Input: dimensioned drawing with shaded views. Units: mm. Origin: part minimum x, y, z. Give positions to 0.01 mm unless a question says otherwise; leave off trailing zeros. Order: outer loops, then holes, each group sorted by start corner. A loop starts at its lowest first (then second) coordinate and runs counter-clockwise, first axis right, second up. Notation, with made-up numbers: M 55.5,2.5 L 60.5,2.5 A7 ccw 60.5,14.5 Z; hole C -22,-38.75 d5. An arc over 180 degrees is marked long. Answer in a Markdown table with one row per item. Add a question column.
(1) Section query B-B, the plane x = 4.85. Return loops of the section in (y, z).
(2) Material intervals for line 1 along Y through (x, z) = (5, 1.7); line 2 along Y through (x, z) = (8.25, 1.45); line 3 along X through (y, z) = (25.5, 2.3), sorted ascending.
(3) Mould query, pull axis X, two halves, no side actions, for the marked faces 1, 2, 3 and 4. Classes: pulls with the +X half, pulls with the -X half, needs draft (parallel to the pull), parting line crosses it, or undercut.
(4) Section query A-A, the plane z = 1.5. Return loops of the section in (x, y).
(5) Section query C-C, the plane x = 2.75. Return loops of the section in (y, z), plus the area to 3 significant figures.
(6) Pin query (flat end, axial travel): P1, Ø1, axis at x = 7.5, z = 0.5, coming from the -Y side; P2, Ø1, axis at x = 7, z = 1, coming from the -Y side; P3, Ø4, axis at x = 7, y = 23, coming from the -Z side. Return the tip coordinate at first contact, or that it passes through.
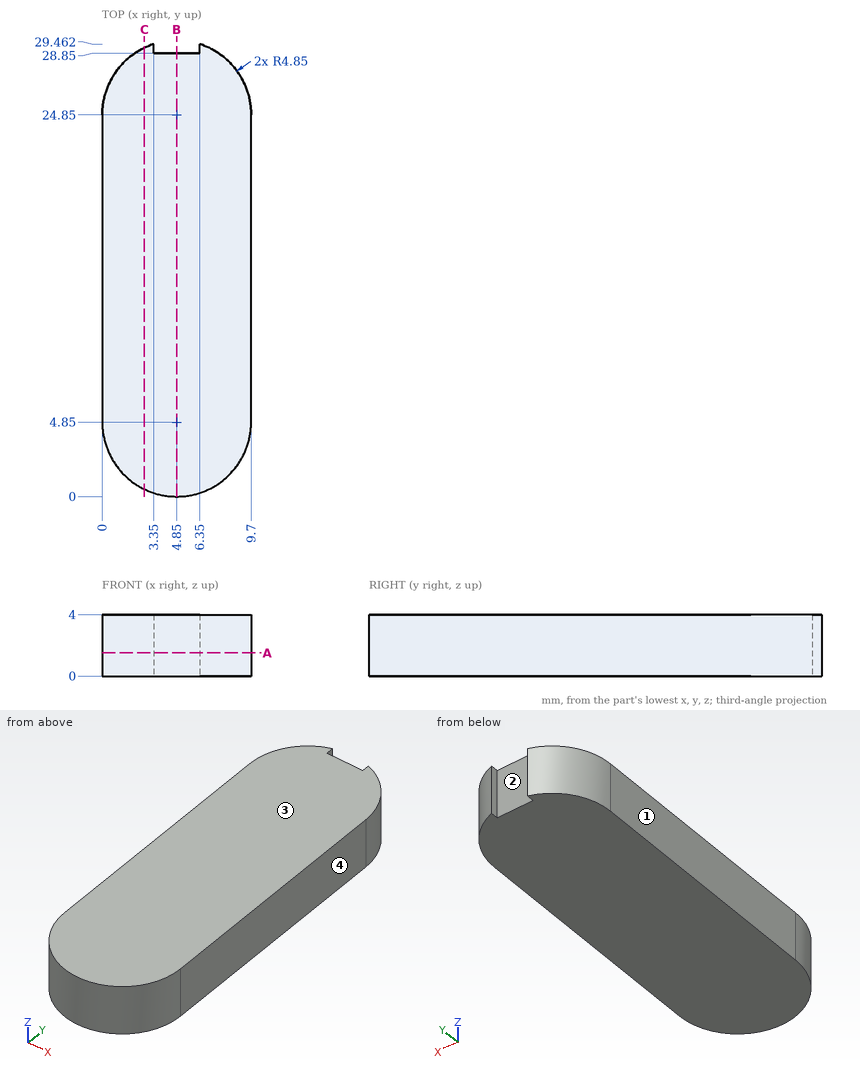
Values follow:
| question | item | result |
|---|---|---|
| 1 | outline | M 0,0 L 28.85,0 L 28.85,4 L 0,4 Z |
| 2 | line 1 | y = 0 to 28.85 |
| 2 | line 2 | y = 1.39 to 28.31 |
| 2 | line 3 | x = 0.04 to 9.66 |
| 3 | face 1 | pulls with the -X half |
| 3 | face 2 | undercut |
| 3 | face 3 | needs draft |
| 3 | face 4 | pulls with the +X half |
| 4 | outline | M 0,4.85 A4.85 ccw 9.7,4.85 L 9.7,24.85 A4.85 ccw 6.35,29.46 L 6.35,28.85 L 3.35,28.85 L 3.35,29.46 A4.85 ccw 0,24.85 Z |
| 5 | outline | M 0.48,0 L 29.22,0 L 29.22,4 L 0.48,4 Z |
| 5 | area | 115 mm² |
| 6 | P1 | stops at y = 0.5 |
| 6 | P2 | stops at y = 0.29 |
| 6 | P3 | stops at z = 0 |
